Job drawing, mm, ordinate dimensions from the low corner. One solid piece. Round coordinates to 2 decimals unless told otherwise and drop trailing zeros. Order: outer loops, then holes, each group sorted by start corner. A loop starts at its lowest first (then second) coordinate and runs counter-clockwise, first axis right, second up. Notation, with made-up numbers: (63, -13) -> (108, -13) arc R15 ccw to (108, -5) -> close; hole circle Ø1 at (-21.5, -8). An arc over 180 degrees is marked (long way). Answer as a JSON object with one key per item and string values. Group by question number.
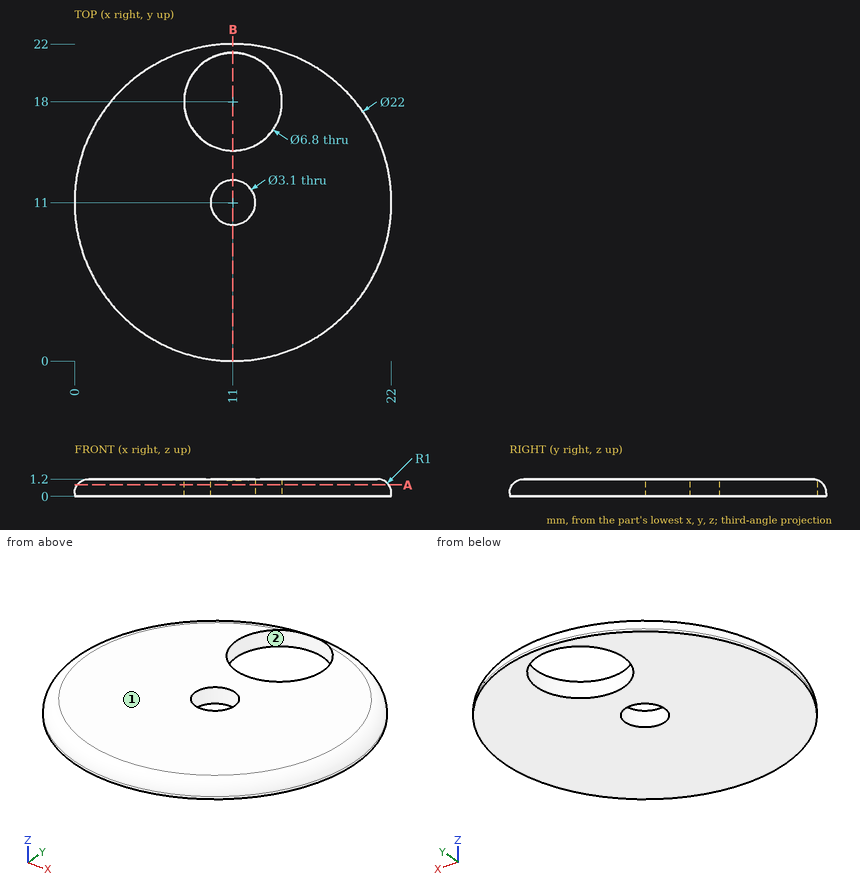
Q1. Band-saw the part on B-B (x = 11). Count the separate pieces of the cut face and the enclosed holes in it, plus the area to 3 significant figures.
Q2. Band-saw the part on A-A (z = 0.8). List the corners of the cut face in (x, y).
Q3. Wall check: line 1 (Y direction, x = 11, z = 0.3); line 2 (Y direction, x = 10.75, z = 0.7); line 3 (X direction, y = 17.75, z = 0.85). Give the ranges that are in metal, low to high. Write a range as [from, to].
Q4. Two-plate mould, pull along Y, no slides. Class the marked faces 1 and 2: +Y half, -Y half, draft (parallel to the pull), parting line (faces both ways), or undercut.
Completed:
{
 "1": {"separate pieces": "3", "enclosed holes": "0", "area": "14.1 mm2"},
 "2": {"outline": "circle Ø21.6 at (11, 11); hole circle Ø6.8 at (11, 18); hole circle Ø3.1 at (11, 11)"},
 "3": {"line 1": "[0.01, 9.45], [12.55, 14.6], [21.4, 21.99]", "line 2": "[0.14, 9.47], [12.53, 14.61], [21.39, 21.86]", "line 3": "[2.62, 7.61], [14.39, 19.38]"},
 "4": {"face 1": "draft", "face 2": "undercut"}
}
